```python
from build123d import *

# Parameters (mm, degrees)
ESQUISSE1_W        = 391
ESQUISSE1_H        = 600
BOSS_EXTRU_1_DEPTH = 10
ESQUISSE2_W        = 50
ESQUISSE2_H        = 50
BOSS_EXTRU_2_DEPTH = 10


with BuildPart() as part:
    # Esquisse1 → Boss.-Extru.1 (new body)
    with BuildSketch(Plane.XY):
        with Locations((-214.094107131, 299.546616829)):
            Rectangle(ESQUISSE1_W, ESQUISSE1_H)
    extrude(amount=-BOSS_EXTRU_1_DEPTH)

    # Esquisse2 → Boss.-Extru.2 (add)
    with BuildSketch(Plane.XY):
        with Locations((-93.594107131, 494.546616829)):
            Rectangle(ESQUISSE2_W, ESQUISSE2_H)
        with Locations((-93.594107131, 104.546616829)):
            Rectangle(ESQUISSE2_W, ESQUISSE2_H)
    extrude(amount=BOSS_EXTRU_2_DEPTH)


solid = part.part
```
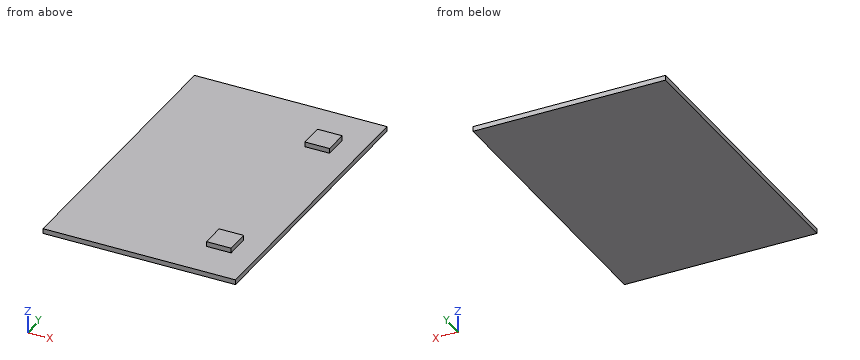
Check sheet for the modelled part. Datum: model origin and axes. Units: mm. Give positions to 0.01 mm unless a question says otherwise; leave off trailing zeros. Write each loop counter-clockwise with the first axis right and the second up, starting at its lowest first coordinate (ties: lowest second). Pieces come first, ordered by that corner, then holes. Notation, with made-up numbers: (82, -16.5) -> (110, -16.5) arc R15 ccw to (110, 11.5) -> close; hole circle Ø3 at (22.25, 39). An arc over 180 degrees is marked (long way). Use CSV: the item, a comma, the result in double quotes. Start each with the question number.
Q1. Cross-section at C-C on y = 297. Enter the section's corners in (x, z), and give its area (3 significant figures).
Q2. Scan lines: line 1 along Y through (x, z) = (-85, 5.25); line 2 along Z through (x, y) = (-133.5, 332.5); line 3 along X through (y, z) = (92, 9). Record each from-to range of solid material in increasing order.
Q3. Cross-section at A-A on z = 3.5. Enter the section's corners in (x, y).
Q4. Cross-section at D-D on x = -172. Enter the section's corners in (y, z), and give its area (3 significant figures).
Q5. Depth check by flat-ended pin: P1, Ø3, axis at x = -100, z = 4.5, coming from the +Y side; P2, Ø5, axis at y = 496, z = 5, coming from the -X side; P3, Ø3, axis at x = -93, z = 6.5, coming from the -Y side; P4, Ø12, axis at y = 240.5, z = 6.5, coming from the +X side. Enter the tip coordinate at first touch or a pass-through.
Q6. Cross-section at B-B on x = -88. Enter the section's corners in (y, z), and give its area (3 significant figures).
Working result:
1,outline,"(-409.59, -10) -> (-18.59, -10) -> (-18.59, 0) -> (-409.59, 0) -> close"
1,area,"3,910 mm^2"
2,line 1,"y = 79.55 to 129.55, 469.55 to 519.55"
2,line 2,"z = -10 to 0"
2,line 3,"x = -118.59 to -68.59"
3,outline,"(-118.59, 79.55) -> (-68.59, 79.55) -> (-68.59, 129.55) -> (-118.59, 129.55) -> close; (-118.59, 469.55) -> (-68.59, 469.55) -> (-68.59, 519.55) -> (-118.59, 519.55) -> close"
4,outline,"(-0.45, -10) -> (599.55, -10) -> (599.55, 0) -> (-0.45, 0) -> close"
4,area,"6,000 mm^2"
5,P1,"stops at y = 519.55"
5,P2,"stops at x = -118.59"
5,P3,"stops at y = 79.55"
5,P4,"passes through"
6,outline,"(-0.45, -10) -> (599.55, -10) -> (599.55, 0) -> (519.55, 0) -> (519.55, 10) -> (469.55, 10) -> (469.55, 0) -> (129.55, 0) -> (129.55, 10) -> (79.55, 10) -> (79.55, 0) -> (-0.45, 0) -> close"
6,area,"7,000 mm^2"
